Geometry: final body of the model. Coordinates: model frame, mm. Coordinates: 2 decimals unless noted, no trailing zeros. Write each loop counter-clockwise with the first axis right and the second up, starting at its lowest first coordinate (ties: lowest second). Pieces come first, ordered by that corner, then holes. Notation, with made-up numbers: (-10.75, -31) -> (42.25, -31) arc R9 cw to (42.25, -18) -> close; hole circle Ø4 at (-12.5, 84.5). An arc over 180 degrees is marked (long way). One line per item, written item: value.
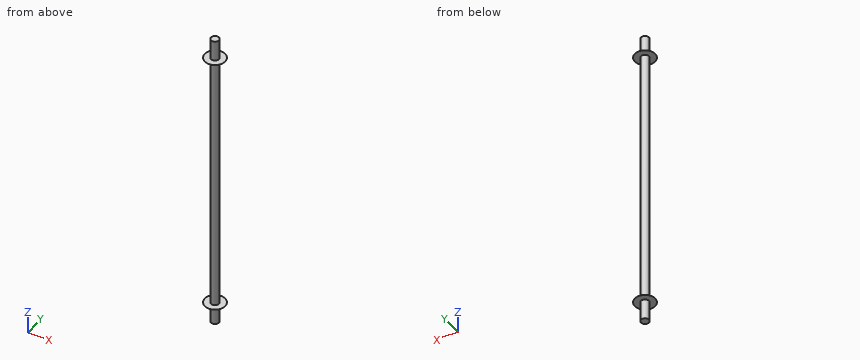
```python
from build123d import *

# Parameters (mm, degrees)
F0_R     = 3.9
F1_DEPTH = 300
F3_R     = 10
F4_DEPTH = 0.001
F6_R     = 10
F7_DEPTH = 0.001


with BuildPart() as f1:
    # F0 (on Top) → F1 (new body)
    with BuildSketch(Plane.XY):
        Circle(F0_R)
    extrude(amount=-F1_DEPTH)

    # F3 (on offset) → F4 (join)
    with BuildSketch(Plane(origin=(0, 0, -280), x_dir=(1, 0, 0), z_dir=(0, 0, -1))):
        Circle(F3_R)
    extrude(amount=-F4_DEPTH)

    # F6 (on offset) → F7 (join)
    with BuildSketch(Plane.XY.offset(-20)):
        Circle(F6_R)
    extrude(amount=-F7_DEPTH)


solid = f1.part
```
(1) Line query: line 1 (Y direction, x = -2, z = -62.5); line 2 (X direction, y = 1.25, z = -152); line 3 (X direction, y = -0.75, z = -16). Output: solid intervals per line, ascending. Write a range as [from, to].
Responses:
line 1: y = [-3.35, 3.35]
line 2: x = [-3.69, 3.69]
line 3: x = [-3.83, 3.83]
(2) First-contact query: pin 1 (3 mm diameter, centred on x = -0.5, z = -39, fed in from -Y); pin 2 (2 mm diameter, centred on x = 5.5, z = -151, fed in from +Y); pin 3 (1 mm diameter, centred on y = -0.5, z = -251.5, fed in from -X); pin 4 (2 mm diameter, centred on x = -7.5, y = 6.5, fed in from -Z). Flat tips, straight axial feed; report the tip coordinate or a pass-through.
Responses:
pin 1: stops at y = -3.9
pin 2: passes through
pin 3: stops at x = -3.9
pin 4: stops at z = -280
(3) Section C-C (z = -225). Return the cut outline in (x, y).
Responses:
outline: circle Ø7.8 at (0, 0)
